Design review of the part built by this model. Coordinates are the model's own, in mm. Coordinates: 2 decimals unless noted, no trailing zeros. Write each loop counter-clockwise with the first axis right and the second up, starting at its lowest first coordinate (ties: lowest second). Pieces come first, ordered by that corner, then holes.
Q1. For probe 1 along X at (y, z) = (3.5, 30); probe 2 along X at (y, z) = (4.5, 39); probe 3 along Z at (x, y) = (117, 2.75), list the stretches that pass through material, from the lowest coordinate up.
Q2. Take a section at B-B (z = 28). Give the boundary of the cut face in (x, y), and give its area (3 significant figures).
Q3. Take a section at A-A (x = 132). Give the boundary of the cut face in (y, z), and give its area (3 significant figures).
Q4. Take a section at C-C (y = 1). Give the boundary of the cut face in (x, z) (3 decimals), and give its area (3 significant figures).
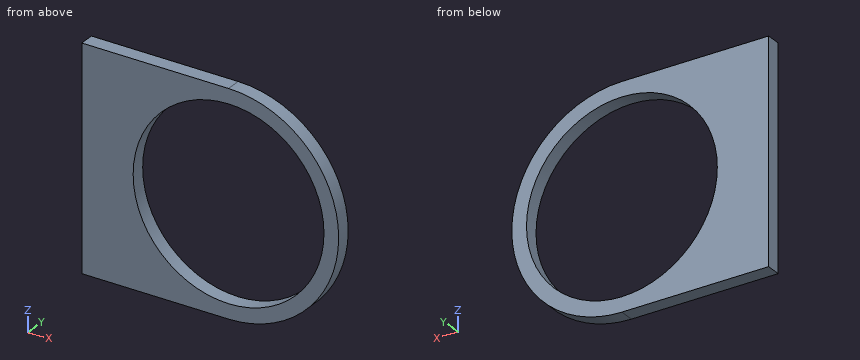
```python
from build123d import *

# Parameters (mm, degrees)
SKETCH2_W           = 111.10281597
SKETCH2_H           = 6.35
BOSS_EXTRUDE1_DEPTH = 95.25
SKETCH3_R           = 41.275
CUT_EXTRUDE2_DEPTH  = 7.35
CUT_EXTRUDE3_DEPTH  = 7.35


with BuildPart() as part:
    # Sketch2 → Boss-Extrude1 (new body)
    with BuildSketch(Plane.XY):
        with Locations((100.171199764, 3.175)):
            Rectangle(SKETCH2_W, SKETCH2_H)
    extrude(amount=BOSS_EXTRUDE1_DEPTH)

    # Sketch3 → Cut-Extrude2 (cut, through all)
    with BuildSketch(Plane(origin=(0, 6.35, 0), x_dir=(1, 0, 0), z_dir=(0, 1, 0))):
        with Locations((108.097607749, -47.625)):
            Circle(SKETCH3_R)
    extrude(amount=-CUT_EXTRUDE2_DEPTH, mode=Mode.SUBTRACT)

    # Sketch4 → Cut-Extrude3 (cut, through all)
    with BuildSketch(Plane(origin=(0, 6.35, 0), x_dir=(1, 0, 0), z_dir=(0, 1, 0))):
        with BuildLine():
            Line((108.097607749, -95.25), (179.051442703, -95.25))
            Line((179.051442703, -95.25), (179.051442703, 0))
            Line((179.051442703, 0), (108.097607749, 0))
            ThreePointArc((108.097607749, 0), (155.722607749, -47.625), (108.097607749, -95.25))
        make_face()
    extrude(amount=-CUT_EXTRUDE3_DEPTH, mode=Mode.SUBTRACT)


solid = part.part
```
Response:
1. probe 1: x = 44.62 to 70.77, 145.42 to 152.34
1. probe 2: x = 44.62 to 67.73, 148.46 to 154.94
1. probe 3: z = 0.84 to 7.32, 87.93 to 94.41
2. outline: (44.62, 0) - (71.79, 0) - (71.79, 6.35) - (44.62, 6.35) - close; (144.41, 0) - (151.49, 0) - (151.49, 6.35) - (144.41, 6.35) - close
2. area: 217 mm2
3. outline: (0, 6.43) - (6.35, 6.43) - (6.35, 13.98) - (0, 13.98) - close; (0, 81.27) - (6.35, 81.27) - (6.35, 88.82) - (0, 88.82) - close
3. area: 95.8 mm2
4. outline: (44.62, 0) - (108.098, 0) arc R47.625 ccw to (108.098, 95.25) - (44.62, 95.25) - close; hole circle Ø82.55 at (108.098, 47.625)
4. area: 4,260 mm2
